```python
from build123d import *

# Parameters (mm, degrees)
BOSS_EXTRUDE1_DEPTH = 20
CUT_EXTRUDE1_DEPTH  = 20
CUT_EXTRUDE2_DEPTH  = 20
SKETCH4_W           = 36.5
SKETCH4_H           = 63
CUT_EXTRUDE3_DEPTH  = 20
FILLET1_R           = 7
FILLET2_R           = 7
SKETCH5_R           = 5
CUT_EXTRUDE4_DEPTH  = 20
CUT_EXTRUDE5_DEPTH  = 20
FILLET3_R           = 7
FILLET4_R           = 7


with BuildPart() as part:
    # Sketch1 → Boss-Extrude1 (new body)
    with BuildSketch(Plane(origin=(0, 0, 0), x_dir=(1, 0, 0), z_dir=(0, 1, 0))):
        Polygon((0, 0), (0, 101), (60, 101), (60, -1.275996113), align=None)
    extrude(amount=BOSS_EXTRUDE1_DEPTH)

    # Sketch2 → Cut-Extrude1 (cut)
    with BuildSketch(Plane(origin=(0, 20, 0), x_dir=(1, 0, 0), z_dir=(0, 1, 0))):
        Polygon((60, 101), (42, 101), (60, 87), align=None)
    extrude(amount=-CUT_EXTRUDE1_DEPTH, mode=Mode.SUBTRACT)

    # Sketch3 → Cut-Extrude2 (cut)
    with BuildSketch(Plane(origin=(0, 20, 0), x_dir=(1, 0, 0), z_dir=(0, 1, 0))):
        Polygon((60, -1.275996113), (46, -0.978263686), (60, 12.724003887), align=None)
        Polygon((10, -0.212666019), (0, 0), (0, 11), align=None)
    extrude(amount=-CUT_EXTRUDE2_DEPTH, mode=Mode.SUBTRACT)

    # Sketch4 → Cut-Extrude3 (cut)
    with BuildSketch(Plane(origin=(0, 20, 0), x_dir=(1, 0, 0), z_dir=(0, 1, 0))):
        with Locations((18.25, 50.5)):
            Rectangle(SKETCH4_W, SKETCH4_H)
    extrude(amount=-CUT_EXTRUDE3_DEPTH, mode=Mode.SUBTRACT)

    # Fillet1
    fillet1_edges = [part.edges().sort_by_distance(p)[0] for p in [
        (36.5, 10, -82),
    ]]
    fillet(fillet1_edges, radius=FILLET1_R)

    # Fillet2
    fillet2_edges = [part.edges().sort_by_distance(p)[0] for p in [
        (36.5, 10, -19),
    ]]
    fillet(fillet2_edges, radius=FILLET2_R)

    # Sketch5 → Cut-Extrude4 (cut)
    with BuildSketch(Plane(origin=(0, 0, -101), x_dir=(-1, 0, 0), z_dir=(0, 0, -1))):
        with Locations((-9.5, 9.5)):
            Circle(SKETCH5_R)
    extrude(amount=-CUT_EXTRUDE4_DEPTH, mode=Mode.SUBTRACT)

    # Sketch7 → Cut-Extrude5 (cut)
    with BuildSketch(Plane(origin=(0, 20, 0), x_dir=(1, 0, 0), z_dir=(0, 1, 0))):
        Polygon((29.5, 82), (40, 82), (40, 19), (0, 19), (0, 82), align=None)
    extrude(amount=-CUT_EXTRUDE5_DEPTH, mode=Mode.SUBTRACT)

    # Fillet3
    fillet3_edges = [part.edges().sort_by_distance(p)[0] for p in [
        (40, 10, -82),
    ]]
    fillet(fillet3_edges, radius=FILLET3_R)

    # Fillet4
    fillet4_edges = [part.edges().sort_by_distance(p)[0] for p in [
        (40, 10, -19),
    ]]
    fillet(fillet4_edges, radius=FILLET4_R)


solid = part.part
```
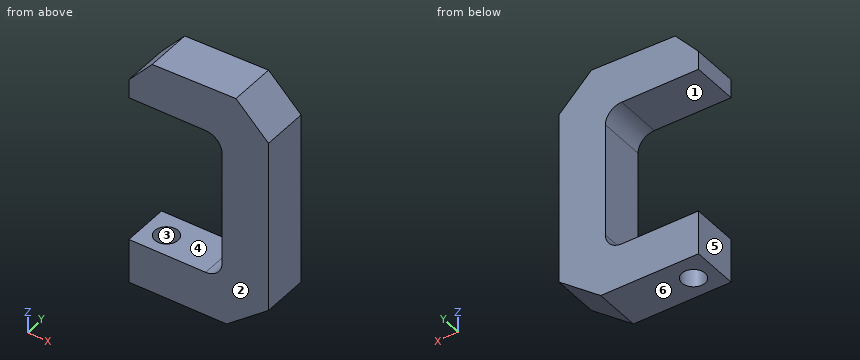
Can you work these out from the model? Positions are in its coordinate system, mm. Face numbers are marked on the shaded views. A direction names the side the tool comes from. Coordinates: 2 decimals unless noted, no trailing zeros. Loops run counter-clockwise (first coordinate to the right, second up) from the corner with the lowest first, then second, coordinate; pieces in that order, holes last.
Item 1: If we mould it in two halves opening along Z, with no side actions, what happens to the marked faces 4, 5 and 6? For each: released by +Z, released by -Z, zero draft, split by the parting line, or undercut.
Answers below:
face 4: undercut
face 5: zero draft
face 6: released by -Z
Item 2: Suppose I cut it at B-B (y = 17). Please give me the cut outline in (x, z), then the cut area to 3 significant figures.
Answers below:
outline: (0, -101) - (42, -101) - (60, -87) - (60, -12.72) - (46, 0.98) - (10, 0.21) - (0, -11) - (0, -19) - (33, -19) arc R7 cw to (40, -26) - (40, -75) arc R7 cw to (33, -82) - (0, -82) - close
area: 3,320 mm2
Item 3: Suppose I cut it at C-C (x = 34). Please give me the cut outline in (y, z), then the cut area to 3 significant figures.
Answers below:
outline: (0, -101) - (20, -101) - (20, -81.93) - (0, -81.93) - close; (0, -19.07) - (20, -19.07) - (20, 0.72) - (0, 0.72) - close
area: 777 mm2
Item 4: I'm going to push flat-ended pins straight in: pin 1 (6 mm diameter, centred on x = 24.5, y = 8, fed in from +Z); pin 2 (5 mm diameter, centred on x = 33, y = 6, fed in from +Z); pin 3 (3 mm diameter, centred on x = 19, y = 10.5, fed in from +Z); pin 4 (8 mm diameter, centred on x = 26, z = -88, fed in from -Y). Where does each tip first touch, or does it pass through?
Answers below:
pin 1: stops at z = 0.58
pin 2: stops at z = 0.75
pin 3: stops at z = 0.44
pin 4: stops at y = 0
Item 5: Please list where these lines run through material, in increasing order: L1, parallel to Y at x = 9.5, z = -87.25; L2, parallel to Z at x = 38.5, y = 14.5; L3, parallel to Z at x = 6, y = 17.25.
Answers below:
L1: y = 0 to 4.5, 14.5 to 20
L2: z = -101 to -79.33, -21.67 to 0.82
L3: z = -101 to -82, -19 to -4.27
Item 6: Suppose I cut it at A-A (y = 9.5). Please give me the cut outline in (x, z), then the cut area to 3 significant figures.
Answers below:
outline: (0, -101) - (4.5, -101) - (4.5, -82) - (0, -82) - close; (0, -19) - (33, -19) arc R7 cw to (40, -26) - (40, -75) arc R7 cw to (33, -82) - (14.5, -82) - (14.5, -101) - (42, -101) - (60, -87) - (60, -12.72) - (46, 0.98) - (10, 0.21) - (0, -11) - close
area: 3,130 mm2
Item 7: Suppose I cut it at D-D (z = -60). Please give me the cut outline in (x, y).
Answers below:
outline: (40, 0) - (60, 0) - (60, 20) - (40, 20) - close
Item 8: Which directions (+Z, -Z, +X, -X, +Y, -Y) give clear straight access to the entire face, cutting with the end or side of a thin tool? Please do the marked faces 1, 2 and 3.
Answers below:
face 1: -X, +Y, -Y
face 2: +Z, -Z, +X, -X, -Y
face 3: -Z
